Read the model definition and answer for the solid it produces. Units are mm, in the model's axes. A direction names the side the tool comes from. Round coordinates to 2 decimals unless told otherwise and drop trailing zeros. Write each loop counter-clockwise with the first axis right and the second up, starting at its lowest first coordinate (ties: lowest second). Pieces come first, ordered by that corner, then holes.
from build123d import *

# Parameters (mm, degrees)
SKICA1_W                 = 72
SKICA1_H                 = 12
SKICA1_R                 = 2
P_IDAT_VYSUNUT_M1_DEPTH  = 4
SKICA2_R                 = 3.5
ODEBRAT_VYSUNUT_M1_DEPTH = 2
SKICA3_W                 = 44
SKICA3_H                 = 12
P_IDAT_VYSUNUT_M2_DEPTH  = 11
SKICA4_W                 = 36
SKICA4_H                 = 12
ODEBRAT_VYSUNUT_M2_DEPTH = 11


with BuildPart() as part:
    # Skica1 → Přidat vysunutím1 (new body)
    with BuildSketch(Plane.XY):
        Rectangle(SKICA1_W, SKICA1_H)
        with Locations((-30, 0)):
            Circle(SKICA1_R, mode=Mode.SUBTRACT)
        with Locations(Location((30, 0, 0), (0, 0, 180))):
            Circle(SKICA1_R, mode=Mode.SUBTRACT)
    extrude(amount=P_IDAT_VYSUNUT_M1_DEPTH)

    # Skica2 → Odebrat vysunutím1 (cut)
    with BuildSketch(Plane.XY.offset(4)):
        with Locations((-30, 0)):
            Circle(SKICA2_R)
        with Locations(Location((30, 0, 0), (0, 0, 180))):
            Circle(SKICA2_R)
    extrude(amount=-ODEBRAT_VYSUNUT_M1_DEPTH, mode=Mode.SUBTRACT)

    # Skica3 → Přidat vysunutím2 (add)
    with BuildSketch(Plane(origin=(0, 0, 0), x_dir=(-1, 0, 0), z_dir=(0, 0, -1))):
        Rectangle(SKICA3_W, SKICA3_H)
    extrude(amount=P_IDAT_VYSUNUT_M2_DEPTH)

    # Skica4 → Odebrat vysunutím2 (cut)
    with BuildSketch(Plane.XY.offset(4)):
        Rectangle(SKICA4_W, SKICA4_H)
    extrude(amount=-ODEBRAT_VYSUNUT_M2_DEPTH, mode=Mode.SUBTRACT)


solid = part.part
Q1. Section C-C (x = -30) is taken. Determine the outline of the cut face in (y, z), then the cut area to 3 significant figures.
Verdict:
outline: (-6, 0) - (-2, 0) - (-2, 2) - (-3.5, 2) - (-3.5, 4) - (-6, 4) - close; (2, 0) - (6, 0) - (6, 4) - (3.5, 4) - (3.5, 2) - (2, 2) - close
area: 26.0 mm2
Q2. Determine the mould class of faces 5 (the cylindrical face through (28.092, -0.601, 0.986)), 6 (the flat face through (36, 0, 2)), 7 (the flat face through (0, -6, -8)) for opening direction Y: pulls with the +Y half, pulls with the -Y half, needs draft (parallel to the pull), parting line crosses it, or undercut.
Verdict:
face 5: undercut
face 6: needs draft
face 7: pulls with the -Y half
Q3. Section B-B (y = 0) is taken. Determine the outline of the cut face in (x, z).
Verdict:
outline: (-36, 0) - (-32, 0) - (-32, 2) - (-33.5, 2) - (-33.5, 4) - (-36, 4) - close; (-28, 0) - (-22, 0) - (-22, -11) - (22, -11) - (22, 0) - (28, 0) - (28, 2) - (26.5, 2) - (26.5, 4) - (18, 4) - (18, -7) - (-18, -7) - (-18, 4) - (-26.5, 4) - (-26.5, 2) - (-28, 2) - close; (32, 0) - (36, 0) - (36, 4) - (33.5, 4) - (33.5, 2) - (32, 2) - close
Q4. Flat-ended cylindrical pins translate along their axes: pin 1 Ø2 at (x, y) = (15, 1.5) entering from +Z; pin 2 Ø3.5 at (y, z) = (2.5, -1.5) entering from +X; pin 3 Ø5 at (x, y) = (-30, 0) entering from +Z; pin 4 Ø3.5 at (y, z) = (-1, -7.5) entering from +X. Find the tip coordinate at first contact, or state that the pin passes through.
Verdict:
pin 1: stops at z = -7
pin 2: stops at x = 36
pin 3: stops at z = 2
pin 4: stops at x = 22
Q5. Straight lines are drawn through the part: probe 1 along Y at (x, z) = (30, 3.1); probe 2 along Y at (x, z) = (-30, 0.75); probe 3 along X at (y, z) = (-3.25, 0.25). For each, find the intervals that lie inside material, in ascending order.
Verdict:
probe 1: y = -6 to -3.5, 3.5 to 6
probe 2: y = -6 to -2, 2 to 6
probe 3: x = -36 to -18, 18 to 36
Q6. Section A-A (z = -3) is taken. Determine the outline of the cut face in (x, y).
Verdict:
outline: (-22, -6) - (-18, -6) - (-18, 6) - (-22, 6) - close; (18, -6) - (22, -6) - (22, 6) - (18, 6) - close
Q7. Section D-D (x = 30.5) is taken. Determine the outline of the cut face in (y, z).
Verdict:
outline: (-6, 0) - (-1.94, 0) - (-1.94, 2) - (-3.46, 2) - (-3.46, 4) - (-6, 4) - close; (1.94, 0) - (6, 0) - (6, 4) - (3.46, 4) - (3.46, 2) - (1.94, 2) - close
Q8. Which of the six approach directions +Z, -Z, +X, -X, +Y, -Y give full straight-line access (tool end or side, diameter ignored) to faces 1 (the flat face through (22, 0, -5)), 2 (the flat face through (28, 2, 2)), 3 (the flat face through (-27.5, 0.1, 0)), 4 (the flat face through (18, 0, -1))?
Verdict:
face 1: -Z, +X, +Y, -Y
face 2: +Z
face 3: -Z, -X, +Y, -Y
face 4: +Z, +Y, -Y
